Part print with two shaded views. Sizes in mm from the minimum x, y, z corner. A direction names the side the tool comes from. Round coordinates to 2 decimals unless told otherwise and drop trailing zeros. Write each loop counter-clockwise with the first axis right and the second up, starting at its lowest first coordinate (ties: lowest second). Pieces come first, ordered by that corner, then holes. Notation, with made-up numbers: (-31, -5) -> (15, -5) arc R8 cw to (15, 7) -> close; hole circle Ø5 at (-20, -4.75). An arc over 180 degrees is marked (long way). Answer in a Markdown table with one row per item.
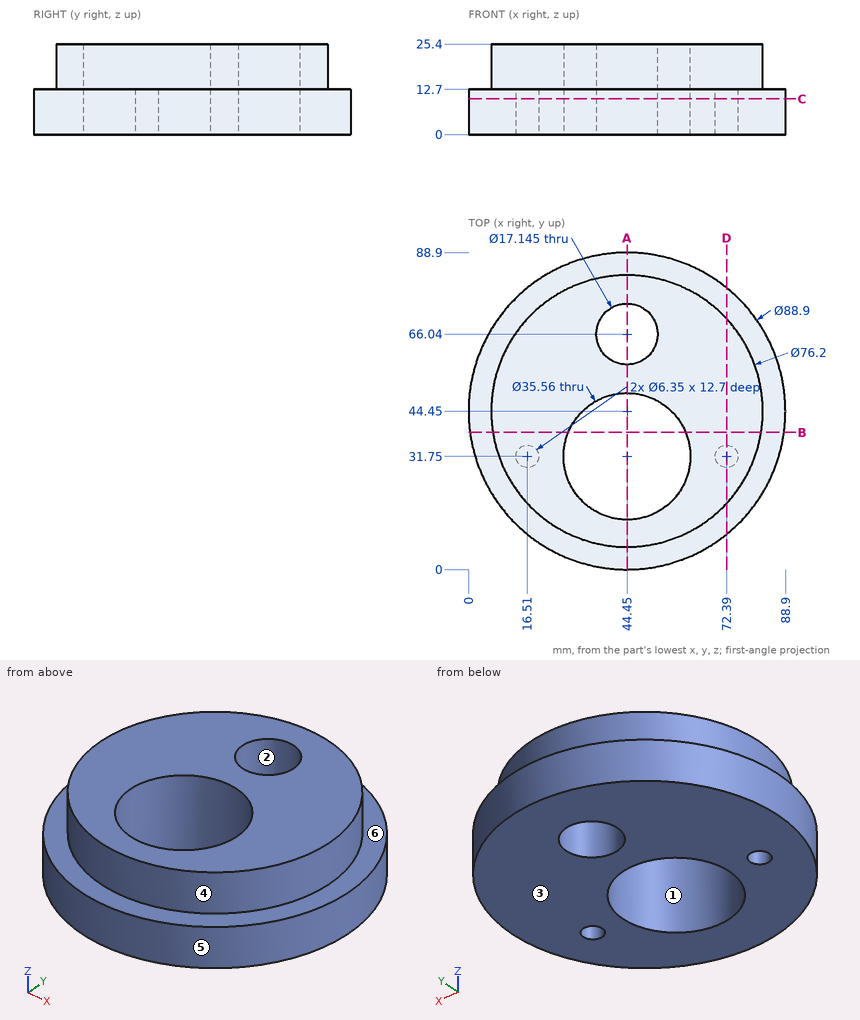
Q1. Saw through at D-D on x = 72.39. Write the cut outline in (y, z) (3 decimals), plus the area to 3 significant figures.
A:
| item | result |
|---|---|
| outline | (9.879, 0) -> (28.575, 0) -> (28.575, 12.7) -> (34.925, 12.7) -> (34.925, 0) -> (79.021, 0) -> (79.021, 12.7) -> (70.353, 12.7) -> (70.353, 25.4) -> (18.547, 25.4) -> (18.547, 12.7) -> (9.879, 12.7) -> close |
| area | 1,460 mm² |
Q2. Drop flat-ended pins along their axis: P1, Ø3, axis at x = 22, y = 11.5, coming from the +Z side; P2, Ø10, axis at y = 32, z = 7, coming from the +X side; P3, Ø10, axis at x = 47.5, z = 13.5, coming from the -Y side. Give the stop position or say it passes through.
A:
| item | result |
|---|---|
| P1 | z = 12.7 |
| P2 | x = 88.27 |
| P3 | y = 0 |
Q3. Two-plate mould, pull along Y, no slides. Class the marked faces 1, 2, 3 and 4: released by +Y, released by -Y, zero draft, split by the parting line, or undercut.
A:
| item | result |
|---|---|
| face 1 | undercut |
| face 2 | undercut |
| face 3 | zero draft |
| face 4 | split by the parting line |
Q4. Wall check: line 1 (Y direction, x = 44.45, z = 19.75); line 2 (X direction, y = 30, z = 12.5); line 3 (Z direction, x = 65, y = 81.5). Give the ranges that are in metal, low to high. Write a range as [from, to].
A:
| item | result |
|---|---|
| line 1 | [6.35, 13.97], [49.53, 57.47], [74.61, 82.55] |
| line 2 | [2.41, 13.86], [19.16, 26.76], [62.14, 69.74], [75.04, 86.49] |
| line 3 | [0, 12.7] |
Q5. Saw through at B-B on y = 38.5. Write the cut outline in (x, z), plus the area to 3 significant figures.
A:
| item | result |
|---|---|
| outline | (0.4, 0) -> (28, 0) -> (28, 25.4) -> (6.82, 25.4) -> (6.82, 12.7) -> (0.4, 12.7) -> close; (60.9, 0) -> (88.5, 0) -> (88.5, 12.7) -> (82.08, 12.7) -> (82.08, 25.4) -> (60.9, 25.4) -> close |
| area | 1,240 mm² |
Q6. Which spindle directions (+Z, -Z, +X, -X, +Y, -Y) get a long thin tool onto all of the face, cutting with end or side? Do the marked faces 5 and 6. Say none if no direction does.
A:
| item | result |
|---|---|
| face 5 | +Z, -Z |
| face 6 | +Z |
Q7. Saw through at A-A on x = 44.45. Write the cut outline in (y, z).
A:
| item | result |
|---|---|
| outline | (0, 0) -> (13.97, 0) -> (13.97, 25.4) -> (6.35, 25.4) -> (6.35, 12.7) -> (0, 12.7) -> close; (49.53, 0) -> (57.47, 0) -> (57.47, 25.4) -> (49.53, 25.4) -> close; (74.61, 0) -> (88.9, 0) -> (88.9, 12.7) -> (82.55, 12.7) -> (82.55, 25.4) -> (74.61, 25.4) -> close |
Q8. Saw through at C-C on z = 10. State how many separate pieces and enclosed holes the cut face has, plus the area to 3 significant figures.
A:
| item | result |
|---|---|
| separate pieces | 1 |
| enclosed holes | 4 |
| area | 4,920 mm² |
